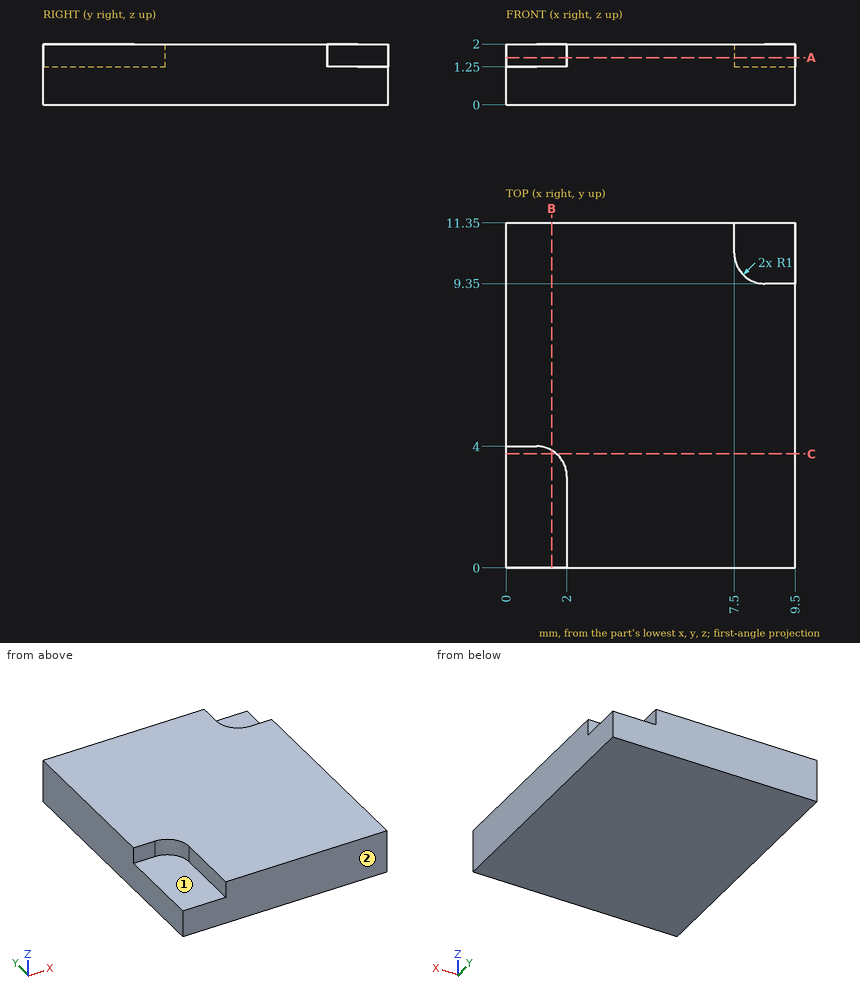
Drawing for the job (mm, zero at the part's lowest x, y, z). A direction names the side the tool comes from. Give positions to 0.01 mm unless a question says otherwise; leave off trailing zeros. Write each loop counter-clockwise with the first axis right and the second up, starting at its lowest first coordinate (ties: lowest second). Pieces come first, ordered by that corner, then holes. Notation, with made-up numbers: (-19, -2.5) - (21, -2.5) arc R12 ccw to (21, 18.5) - close; hole circle Ø9 at (35.25, 59.5). An arc over 180 degrees is marked (long way). Answer as CSV lines item,"result".
Q1. Band-saw the part on C-C (y = 3.75). Give the cut face in (x, z), and give its area (3 significant figures).
Result set:
outline,"(0, 0) - (9.5, 0) - (9.5, 2) - (1.66, 2) - (1.66, 1.25) - (0, 1.25) - close"
area,"17.8 mm²"
Q2. Drill centre lines: line 1 (X direction, y = 10.5, z = 1.9); line 2 (Z direction, x = 8.5, y = 10.25); line 3 (Y direction, x = 8.75, z = 1.75). Where is each one in solid material? Low to high. Write a range as from..to.
Result set:
line 1,"0..7.5"
line 2,"0..1.25"
line 3,"0..9.35"
Q3. Flat gauge pins, fed straight in: pin 1 Ø0.6 at (x, z) = (0.5, 1.5) entering from -Y; pin 2 Ø1 at (x, y) = (0.5, 2.5) entering from +Z. Where does each tip first touch, or does it go through?
Result set:
pin 1,"y = 0"
pin 2,"z = 1.25"
Q4. Band-saw the part on A-A (z = 1.55). Give the cut face in (x, y).
Result set:
outline,"(0, 4) - (1, 4) arc R1 cw to (2, 3) - (2, 0) - (9.5, 0) - (9.5, 9.35) - (8.5, 9.35) arc R1 cw to (7.5, 10.35) - (7.5, 11.35) - (0, 11.35) - close"
Q5. Band-saw the part on B-B (x = 1.5). Give the cut face in (y, z), and give its area (3 significant figures).
Result set:
outline,"(0, 0) - (11.35, 0) - (11.35, 2) - (3.87, 2) - (3.87, 1.25) - (0, 1.25) - close"
area,"19.8 mm²"
Q6. 3-axis set-ups, long thin cutter, end or side, ignore diameter. For the marked faces 1 and 2: which of +Z, -Z, +X, -X, +Y, -Y reach the whole face in a straight line?
Result set:
face 1,"+Z, -X, -Y"
face 2,"+Z, -Z, +X, -X, -Y"
